```python
from build123d import *

# Parameters (mm, degrees)
ESBO_O1_W                = 55
ESBO_O1_H                = 25
RESSALTO_EXTRUS_O1_DEPTH = 354.77
CASCA1_T                 = -5
ESBO_O3_W                = 4
ESBO_O3_H                = 30
CORTE_EXTRUS_O1_DEPTH    = 360.564671374


with BuildPart() as part:
    # Esboço1 → Ressalto-extrusão1 (new body)
    with BuildSketch(Plane(origin=(0, 0, 0), x_dir=(0, 0, -1), z_dir=(1, 0, 0))):
        with Locations((27.5, 12.5)):
            Rectangle(ESBO_O1_W, ESBO_O1_H)
    extrude(amount=RESSALTO_EXTRUS_O1_DEPTH)

    # Casca1
    casca1_openings = [part.faces().sort_by_distance(p)[0] for p in [
        (177.385, 25, -27.5),
    ]]
    offset(amount=CASCA1_T, openings=casca1_openings, kind=Kind.INTERSECTION)

    # Esboço3 → Corte-extrusão1 (cut, through all)
    with BuildSketch(Plane(origin=(0, 5, 0), x_dir=(1, 0, 0), z_dir=(0, 1, 0))):
        with Locations((347.77, 27.5)):
            Rectangle(ESBO_O3_W, ESBO_O3_H)
    extrude(amount=-CORTE_EXTRUS_O1_DEPTH, mode=Mode.SUBTRACT)


solid = part.part
```
Can you work these out from the model? Positions are in its coordinate system, mm. A direction names the side the tool comes from. Round coordinates to 2 decimals unless told otherwise and drop trailing zeros. Loops run counter-clockwise (first coordinate to the right, second up) from the corner with the lowest first, then second, coordinate; pieces in that order, holes last.
Item 1: Suppose I cut it at B-B, the plane y = 18. Write out the boundary of the cut face in (x, z).
Item 2: Please list where these lines run through material, in increasing order: L1, parallel to X at y = 21.75, z = -30; L2, parallel to Z at x = 246.5, y = 21.5; L3, parallel to Y at x = 67.5, z = -16.5.
Item 3: Suppose I cut it at D-D, the plane z = -9.5. Write out the boundary of the cut face in (x, y), then the cut area to 3 significant figures.
Item 4: Suppose I cut it at A-A, the plane z = -34. Write out the boundary of the cut face in (x, y).
Item 5: Will these pins go through, and if not, where does the flat tip stop? pin 1 Ø4.5 at (x, y) = (347.5, 2) entering from +Z; pin 2 Ø12 at (x, z) = (200, -38.5) entering from +Y.
Item 6: Which directions (+Z, -Z, +X, -X, +Y, -Y) give clear straight access to the entire face, cutting with the end or side of a thin tool? Please do faces 4 (the flat face through (175, 15, -50)), 5 (the flat face through (0, 13, -27)).
Item 7: Suppose I cut it at C-C, the plane x = 300.5. Write out the boundary of the cut face in (y, z), then the cut area to 3 significant figures.
Item 8: If we mould it in two halves opening along Z, with no side actions, what happens to faces 1 (the flat face through (175, 12, -55)), 2 (the flat face through (349.77, 13, -27)), 3 (the flat face through (177, 25, -3))? For each: +Z half, -Z half, draft (parallel to the pull), parting line (faces both ways), or undercut.
Reported:
1. outline: (0, -55) - (354.77, -55) - (354.77, 0) - (0, 0) - close; hole (5, -50) - (349.77, -50) - (349.77, -5) - (5, -5) - close
2. L1: x = 0 to 5, 349.77 to 354.77
2. L2: z = -55 to -50, -5 to 0
2. L3: y = 0 to 5
3. outline: (0, 0) - (354.77, 0) - (354.77, 25) - (349.77, 25) - (349.77, 5) - (5, 5) - (5, 25) - (0, 25) - close
3. area: 1,970 mm2
4. outline: (0, 0) - (345.77, 0) - (345.77, 5) - (5, 5) - (5, 25) - (0, 25) - close; (349.77, 0) - (354.77, 0) - (354.77, 25) - (349.77, 25) - close
5. pin 1: stops at z = 0
5. pin 2: stops at y = 5
6. face 4: +Y
6. face 5: +Z, -Z, -X, +Y, -Y
7. outline: (0, -55) - (25, -55) - (25, -50) - (5, -50) - (5, -5) - (25, -5) - (25, 0) - (0, 0) - close
7. area: 475 mm2
8. face 1: -Z half
8. face 2: undercut
8. face 3: draft
